Autodesk Inventor part; units mm, degrees
ref_plane "YZ Plane" through (0, 0, 0) normal (1, 0, 0) x (0, 1, 0)
ref_plane "XZ Plane" through (0, 0, 0) normal (0, 1, 0) x (-1, 0, 0)
ref_plane "XY Plane" through (0, 0, 0) normal (0, 0, 1) x (1, 0, 0)
sketch "Sketch1" plane through (0, 0, 0) normal (0, 0, 1) x (1, 0, 0)
  line L0 (0, 0) -> (-7, 0) construction
  line L1 (0, 4.35) -> (-7, 4.35)
  line L2 (-7, -4.35) -> (0, -4.35)
  arc A0 (0, -4.35) -> (0, 4.35) centre (0, 0) ccw
  arc A1 (-7, 4.35) -> (-7, -4.35) centre (-7, 0) ccw
  line L3 (-7, 3.6) -> (0, 3.6)
  arc A2 (0, -3.6) -> (0, 3.6) centre (0, 0) ccw
  line L4 (0, -3.6) -> (-7, -3.6)
  arc A3 (-7, 3.6) -> (-7, -3.6) centre (-7, 0) ccw
  line L5 (0, -4.35) -> (19.2, -4.35)
  line L6 (20, -3.55) -> (20, -3.15)
  line L7 (19.2, -2.35) -> (3.6606, -2.35)
  circle A4 centre (18.8, -3.35) radius 1
  arc A5 (20, -3.15) -> (19.2, -2.35) centre (19.2, -3.15) ccw
  arc A6 (19.2, -4.35) -> (20, -3.55) centre (19.2, -3.55) ccw
  arc A7 (16.5087, -4.35) -> (16.5087, -2.35) centre (18.8, -3.35) ccw
  line L8 (18.8, -3.35) -> (5.3494, -3.35) construction
  point P0 (-3.5, 0)
  point P1 (20, -4.35)
  point P2 (20, -2.35)
  dimension "d0" = 7
  dimension "d1" = 8.7
  dimension "d5" = 3.6
  dimension "d6" = 2
  dimension "d7" = 2
  dimension "d8" = 20
  dimension "d9" = 1.2
  dimension "d10" = 0.8
  dimension "d13" = 5
  dimension "d14" = 1
extrude "Extrusion1" add sketch "Sketch1" along normal blind 1 contours A0 L2 A1 L1 | L7 A4 L5 A0 | A7 L5 A6 L6 A5 L7 | L7 A5 L6 A6 L5 A4 | L3 A2 L4 A3
extrude "Extrusion2" add sketch "Sketch1" along normal blind 2 from surface at 1 contours L3 A2 L4 A3
properties part number "tappino tpu" material "Thermoplastic Resin"
Part model, mm, in its own coordinate system. A direction names the side the tool comes from. Coordinates: 2 decimals unless noted, no trailing zeros. Loops run counter-clockwise (first coordinate to the right, second up) from the corner with the lowest first, then second, coordinate; pieces in that order, holes last. Notation, with made-up numbers: (70.5, -12) - (75.5, -12) arc R12 cw to (75.5, 7) - close; hole circle Ø9 at (76.5, 16). An arc over 180 degrees is marked (long way). Write each question's results on one line, items separated by ' | '. Start each with the question number.
Q1. Two-plate mould, pull along X, no slides. Class faces 4 (the flat face through (-4, 0, 3)), 5 (the cylindrical face through (21.3, -3.3, 0.5)), 6 (the cylindrical face through (-11.35, -0.1, 0.49)): +X half, -X half, draft (parallel to the pull), parting line (faces both ways), or undercut.
Q2. Slice it at B-B on x = -4.5. Give the cut face in (y, z).
Q3. Drop flat-ended pins along their axis: pin 1 Ø6 at (x, y) = (15.5, -2.5) entering from +Z; pin 2 Ø0.5 at (x, z) = (4.5, 0.5) entering from -Y; pin 3 Ø0.6 at (x, z) = (-2.5, 2) entering from -Y. Give the stop position or say it passes through.
Q4. Which spindle directions (+Z, -Z, +X, -X, +Y, -Y) get a long thin tool onto all of the face, cutting with end or side? Do faces 1 (the cylindrical face through (3.6, 0.1, 2)), 2 (the flat face through (4.6, -4.35, 0.5)), 3 (the flat face through (6, -3, 1)). Say none if no direction does.
Q5. Slice it at A-A on z = 0.6. Give the cut face in (x, y), and give its area (3 significant figures).
Q6. Probe line 1 along Y through (x, z) = (18.8, 0.25); line 2 along Y through (x, z) = (-3, 0.45); line 3 along X through (y, z) = (-3.35, 0.5). List the from-to ranges inside material, lowest first.
Q7. Slice it at C-C on y = -1.75. Give the cut face in (x, z), and give its area (3 significant figures).
Q8. Slice it at D-D on y = 0. Give the cut face in (x, z), and give its area (3 significant figures).
Answer:
1) face 4: draft | face 5: undercut | face 6: -X half
2) outline: (-4.35, 0) - (4.35, 0) - (4.35, 1) - (3.6, 1) - (3.6, 3) - (-3.6, 3) - (-3.6, 1) - (-4.35, 1) - close
3) pin 1: stops at z = 1 | pin 2: stops at y = -4.35 | pin 3: stops at y = -3.6
4) face 1: +Z, +X | face 2: +Z, -Z, -X, -Y | face 3: +Z
5) outline: (-7, -4.35) - (16.51, -4.35) arc R2.5 ccw (long way) to (16.51, -2.35) - (3.66, -2.35) arc R4.35 ccw to (0, 4.35) - (-7, 4.35) arc R4.35 ccw to start; hole circle Ø2 at (18.8, -3.35) | area: 164 mm2
6) line 1: y = -5.85 to -4.35, -2.35 to -0.85 | line 2: y = -4.35 to 4.35 | line 3: x = -9.77 to 17.8, 19.8 to 21.3
7) outline: (-10.98, 0) - (3.98, 0) - (3.98, 1) - (3.15, 1) - (3.15, 3) - (-10.15, 3) - (-10.15, 1) - (-10.98, 1) - close; (16.88, 0) - (20.72, 0) - (20.72, 1) - (16.88, 1) - close | area: 45.4 mm2
8) outline: (-11.35, 0) - (4.35, 0) - (4.35, 1) - (3.6, 1) - (3.6, 3) - (-10.6, 3) - (-10.6, 1) - (-11.35, 1) - close | area: 44.1 mm2
